Read the model definition and answer for the solid it produces. Units are mm, in the model's axes. Face numbers are marked on the shaded views. A direction names the side the tool comes from. Give positions to 0.01 mm unless a question says otherwise; leave off trailing zeros. Loops run counter-clockwise (first coordinate to the right, second up) from the corner with the lowest first, then second, coordinate; pieces in that order, holes last. Notation, with made-up numbers: (-19.75, 78.25) - (4.25, 78.25) arc R20 cw to (4.25, 92.25) - close; hole circle Ø9 at (70, 20). An arc over 180 degrees is marked (long way). Use a Markdown table: item, result. Add a question column.
Item 1: A cutting plane is placed at A-A (y = -280). Give the number of separate pieces and of enclosed holes in the cut face, plus the area to 3 significant figures.
Item 2: A cutting plane is placed at C-C (x = 368.5). Determine the outline of the cut face in (y, z).
Item 3: Each of these flat-tipped pins is pushed along its axis until it touches: P1, Ø24, axis at y = -280, z = 130, coming from the -X side; P2, Ø8, axis at x = 24, z = 21, coming from the -Y side; P3, Ø3, axis at x = 286.5, z = -45, coming from the -Y side; P4, Ø18, axis at y = -534.5, z = 131.5, coming from the +X side. Where does it stop, or does it pass through?
Item 4: Consider probe 1 along Y at (x, z) = (386, 130); probe 2 along Y at (x, z) = (308, 5.5); probe 3 along Z at (x, y) = (302, -409.5). Determine where each line is inside the solid, lowest interval first. Write a range as [from, to].
Item 5: A cutting plane is placed at B-B (x = 274.5). Determine the outline of the cut face in (y, z), plus the area to 3 significant figures.
Item 6: For a pull along Z with two mould halves and no side action, classify the marked faces 1, 2 and 3 as +Z half, -Z half, draft (parallel to the pull), parting line (faces both ways), or undercut.
Item 7: Which of the six approach directions +Z, -Z, +X, -X, +Y, -Y give full straight-line access (tool end or side, diameter ignored) to the marked faces 4, 5 and 6?
from build123d import *

# Parameters (mm, degrees)
SKETCH2_R           = 145
SKETCH2_R_2         = 105
SKETCH6_R           = 15
BOSS_EXTRUDE1_DEPTH = 50
SKETCH7_R           = 105
CUT_EXTRUDE1_DEPTH  = 50
SKETCH9_W           = 360
SKETCH9_H           = 360
SKETCH9_R           = 15
BOSS_EXTRUDE3_DEPTH = 50
SKETCH10_R          = 30
CUT_EXTRUDE3_DEPTH  = 10
SKETCH11_R          = 30
CUT_EXTRUDE4_DEPTH  = 10
FILLET2_R           = 20
FILLET3_R           = 10
SKETCH12_R          = 105
CUT_EXTRUDE5_DEPTH  = 50
CHAMFER2_SIZE       = 10


with BuildPart() as part:
    # Sweep1: sweep along a path in Sketch4
    with BuildLine(Plane.XY) as sweep1_path:
        Line((0, 0), (0, -150))
        ThreePointArc((0, -150), (76.152236891, -333.847763109), (260, -410))
        Line((260, -410), (410, -410))
    # Sketch2 → Sweep1 (sweep)
    with BuildSketch(Plane(origin=(0, 0, 0), x_dir=(1, 0, 0), z_dir=(0, 1, 0))):
        Circle(SKETCH2_R)
        Circle(SKETCH2_R_2, mode=Mode.SUBTRACT)
    sweep(path=sweep1_path.line)

    # Sketch6 → Boss-Extrude1 (add)
    with BuildSketch(Plane(origin=(0, 0, 0), x_dir=(1, 0, 0), z_dir=(0, 1, 0))):
        with BuildLine():
            Line((-160, 180), (160, 180))
            ThreePointArc((160, 180), (174.142135624, 174.142135624), (180, 160))
            Line((180, 160), (180, -160))
            ThreePointArc((180, -160), (174.142135624, -174.142135624), (160, -180))
            Line((160, -180), (-160, -180))
            ThreePointArc((-160, -180), (-174.142135624, -174.142135624), (-180, -160))
            Line((-180, -160), (-180, 160))
            ThreePointArc((-180, 160), (-174.142135624, 174.142135624), (-160, 180))
        make_face()
        with Locations(Location((-130, 130, 0), (0, 0, 270))):
            Circle(SKETCH6_R, mode=Mode.SUBTRACT)
        with Locations(Location((130, 130, 0), (0, 0, 270))):
            Circle(SKETCH6_R, mode=Mode.SUBTRACT)
        with Locations(Location((130, -130, 0), (0, 0, 270))):
            Circle(SKETCH6_R, mode=Mode.SUBTRACT)
        with Locations(Location((-130, -130, 0), (0, 0, 270))):
            Circle(SKETCH6_R, mode=Mode.SUBTRACT)
    extrude(amount=-BOSS_EXTRUDE1_DEPTH)

    # Sketch7 → Cut-Extrude1 (cut)
    with BuildSketch(Plane(origin=(0, -50, 0), x_dir=(-1, 0, 0), z_dir=(0, -1, 0))):
        with Locations(Location((0, 0, 0), (0, 0, 90))):
            Circle(SKETCH7_R)
    extrude(amount=-CUT_EXTRUDE1_DEPTH, mode=Mode.SUBTRACT)

    # Sketch9 → Boss-Extrude3 (add)
    with BuildSketch(Plane(origin=(410, 0, 0), x_dir=(0, 0, -1), z_dir=(1, 0, 0))):
        with Locations((0, -410)):
            Rectangle(SKETCH9_W, SKETCH9_H)
        with Locations((-130, -280)):
            Circle(SKETCH9_R, mode=Mode.SUBTRACT)
        with Locations((-130, -540)):
            Circle(SKETCH9_R, mode=Mode.SUBTRACT)
        with Locations((130, -540)):
            Circle(SKETCH9_R, mode=Mode.SUBTRACT)
        with Locations((130, -280)):
            Circle(SKETCH9_R, mode=Mode.SUBTRACT)
    extrude(amount=-BOSS_EXTRUDE3_DEPTH)

    # Sketch10 → Cut-Extrude3 (cut)
    with BuildSketch(Plane(origin=(0, 0, 0), x_dir=(1, 0, 0), z_dir=(0, 1, 0))):
        with Locations(Location((-130, 130, 0), (0, 0, 270))):
            Circle(SKETCH10_R)
        with Locations(Location((130, 130, 0), (0, 0, 270))):
            Circle(SKETCH10_R)
        with Locations(Location((130, -130, 0), (0, 0, 270))):
            Circle(SKETCH10_R)
        with Locations(Location((-130, -130, 0), (0, 0, 270))):
            Circle(SKETCH10_R)
    extrude(amount=-CUT_EXTRUDE3_DEPTH, mode=Mode.SUBTRACT)

    # Sketch11 → Cut-Extrude4 (cut)
    with BuildSketch(Plane(origin=(410, 0, 0), x_dir=(0, 0, -1), z_dir=(1, 0, 0))):
        with Locations((-130, -280)):
            Circle(SKETCH11_R)
        with Locations((130, -280)):
            Circle(SKETCH11_R)
        with Locations((-130, -540)):
            Circle(SKETCH11_R)
        with Locations((130, -540)):
            Circle(SKETCH11_R)
    extrude(amount=-CUT_EXTRUDE4_DEPTH, mode=Mode.SUBTRACT)

    # Fillet2
    fillet2_edges = [part.edges().sort_by_distance(p)[0] for p in [
        (385, -230, -180),
        (385, -590, -180),
        (385, -590, 180),
        (385, -230, 180),
    ]]
    fillet(fillet2_edges, radius=FILLET2_R)

    # Fillet3
    fillet3_edges = [part.edges().sort_by_distance(p)[0] for p in [
        (-145, -50, 0),
        (360, -555, 0),
    ]]
    fillet(fillet3_edges, radius=FILLET3_R)

    # Sketch12 → Cut-Extrude5 (cut)
    with BuildSketch(Plane(origin=(410, 0, 0), x_dir=(0, 0, -1), z_dir=(1, 0, 0))):
        with Locations((0, -411.649373871)):
            Circle(SKETCH12_R)
    extrude(amount=-CUT_EXTRUDE5_DEPTH, mode=Mode.SUBTRACT)

    # Chamfer2
    chamfer2_edges = [part.edges().sort_by_distance(p)[0] for p in [
        (410, -411.649373871, 105),
        (0, 0, 105),
    ]]
    chamfer(chamfer2_edges, length=CHAMFER2_SIZE)


solid = part.part
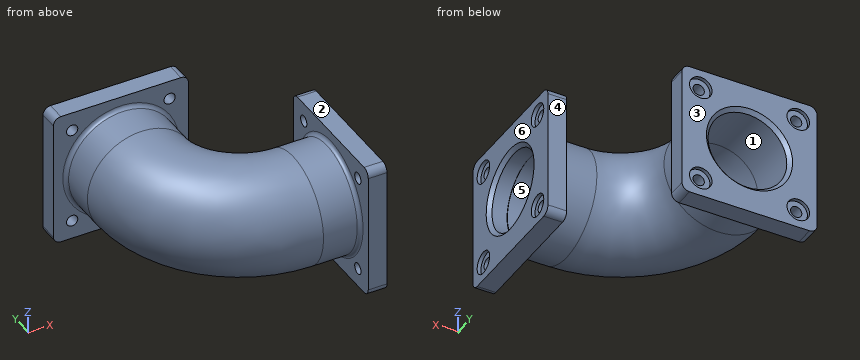
Geometry says:
| question | item | result |
|---|---|---|
| 1 | separate pieces | 3 |
| 1 | enclosed holes | 1 |
| 1 | area | 71,700 mm² |
| 2 | outline | (-590, -160) arc R20 ccw to (-570, -180) - (-250, -180) arc R20 ccw to (-230, -160) - (-230, 160) arc R20 ccw to (-250, 180) - (-570, 180) arc R20 ccw to (-590, 160) - close; hole circle Ø30 at (-540, -130); hole circle Ø30 at (-540, 130); hole circle Ø210 at (-411.65, 0); hole circle Ø30 at (-280, -130); hole circle Ø30 at (-280, 130) |
| 3 | P1 | x = -59.41 |
| 3 | P2 | y = -480.18 |
| 3 | P3 | y = -548.32 |
| 3 | P4 | through |
| 4 | probe 1 | [-590, -555], [-525, -295], [-265, -230] |
| 4 | probe 2 | [-554.9, -514.86], [-305.14, -265.1] |
| 4 | probe 3 | [-145, -105], [105, 145] |
| 5 | outline | circle Ø290 at (-410, 0); hole circle Ø210 at (-410, 0) |
| 5 | area | 31,400 mm² |
| 6 | face 1 | undercut |
| 6 | face 2 | +Z half |
| 6 | face 3 | draft |
| 7 | face 4 | +Z, -Z, +X, +Y |
| 7 | face 5 | none |
| 7 | face 6 | +Z, -Z, +X, +Y, -Y |
